```python
from build123d import *

# Parameters (mm, degrees)
SKETCH8_W           = 84.5
SKETCH8_H           = 12
SKETCH8_R           = 2.456134815
BOSS_EXTRUDE4_DEPTH = 8
SKETCH9_R           = 3.5
CUT_EXTRUDE3_DEPTH  = 2
SKETCH10_W          = 6
SKETCH10_H          = 12
BOSS_EXTRUDE5_DEPTH = 48
SKETCH11_W          = 8
SKETCH11_H          = 3.4
BOSS_EXTRUDE6_DEPTH = 35
SKETCH12_R          = 2
CUT_EXTRUDE4_DEPTH  = 35
SKETCH13_R          = 1.310160124
CUT_EXTRUDE5_DEPTH  = 10


with BuildPart() as part:
    # Sketch8 → Boss-Extrude4 (new body)
    with BuildSketch(Plane.XY):
        with Locations((17.439173688, 7.621093459)):
            Rectangle(SKETCH8_W, SKETCH8_H)
        with Locations((-18.810826312, 7.621093459)):
            Circle(SKETCH8_R, mode=Mode.SUBTRACT)
        with Locations((15.689173688, 7.621093459)):
            Circle(SKETCH8_R, mode=Mode.SUBTRACT)
    extrude(amount=BOSS_EXTRUDE4_DEPTH)

    # Sketch9 → Cut-Extrude3 (cut)
    with BuildSketch(Plane(origin=(0, 0, 0), x_dir=(-1, 0, 0), z_dir=(0, 0, -1))):
        with Locations((-15.689173688, 7.621093459)):
            Circle(SKETCH9_R)
        with Locations((18.810826312, 7.621093459)):
            Circle(SKETCH9_R)
    extrude(amount=-CUT_EXTRUDE3_DEPTH, mode=Mode.SUBTRACT)

    # Sketch10 → Boss-Extrude5 (add)
    with BuildSketch(Plane.XY.offset(8)):
        with Locations((56.689173688, 7.621093459)):
            Rectangle(SKETCH10_W, SKETCH10_H)
    extrude(amount=BOSS_EXTRUDE5_DEPTH)

    # Sketch11 → Boss-Extrude6 (add)
    with BuildSketch(Plane(origin=(59.689173688, 0, 0), x_dir=(0, 0, -1), z_dir=(1, 0, 0))):
        with Locations((-4, 3.321093459)):
            Rectangle(SKETCH11_W, SKETCH11_H)
        with Locations((-52, 3.321093459)):
            Rectangle(SKETCH11_W, SKETCH11_H)
    extrude(amount=BOSS_EXTRUDE6_DEPTH)

    # Sketch12 → Cut-Extrude4 (cut)
    with BuildSketch(Plane(origin=(0, 5.021093459, 0), x_dir=(1, 0, 0), z_dir=(0, 1, 0))):
        with Locations(Location((72.689173688, -3.25, 0), (0, 0, 180))):
            Circle(SKETCH12_R)
        with Locations(Location((82.689173688, -3.25, 0), (0, 0, 180))):
            Circle(SKETCH12_R)
        with Locations(Location((72.689173688, -52.75, 0), (0, 0, 180))):
            Circle(SKETCH12_R)
        with Locations(Location((82.689173688, -52.75, 0), (0, 0, 180))):
            Circle(SKETCH12_R)
    extrude(amount=-CUT_EXTRUDE4_DEPTH, mode=Mode.SUBTRACT)

    # Sketch13 → Cut-Extrude5 (cut)
    with BuildSketch(Plane(origin=(0, 0, 0), x_dir=(-1, 0, 0), z_dir=(0, 0, -1))):
        with Locations((1.505343306, 7.621093459)):
            Circle(SKETCH13_R)
    extrude(amount=-CUT_EXTRUDE5_DEPTH, mode=Mode.SUBTRACT)


solid = part.part
```
Here's how the part is built. I have some questions about the finished solid (model axes, mm). A direction names the side the tool comes from. Coordinates: 2 decimals unless noted, no trailing zeros. Write each loop counter-clockwise with the first axis right and the second up, starting at its lowest first coordinate (ties: lowest second). Pieces come first, ordered by that corner, then holes. Notation, with made-up numbers: (60.5, 0.5) -> (95.5, 0.5) arc R15 cw to (95.5, 20.5) -> close; hole circle Ø7 at (-35, 35). An arc over 180 degrees is marked (long way). Use a Markdown table: item, result. Add a question column.
(1) If we section it at B-B, the plane z = 3.25: Write out the boundary of the cut face in (x, y), and give its area (3 significant figures).
(2) For faces 5 (the cylindrical face through (12.35, 8.67, 0.99)), 6 (the flat face through (77, 5.021, 52)), 7 (the flat face through (77, 3, 48)), 8 (the flat face through (53.689, 8, 32)), which set-ups out of +Z, -Z, +X, -X, +Y, -Y let a thin tool reach every point of the face, with its end or its side?
(3) I'm going to push flat-ended pins straight in: P1, Ø6, axis at y = 5.5, z = 28, coming from the -X side; P2, Ø2.5, axis at x = 78, z = 3, coming from the +Y side; P3, Ø3.5, axis at x = 8.5, y = 8, coming from the +Z side. Where does each tip first touch, or does it pass through?
(4) If we section it at C-C, the plane x = 65.5: Write out the boundary of the cut face in (y, z).
(5) We'd pull the mould along X, two halves only. Please class faces 1 (the flat face through (94.689, 3, 4)), 2 (the cylindrical face through (-22.15, 8.67, 0.99)), 3 (the flat face through (-24.811, 8, 4)), 4 (the flat face through (21, 8, 0)): +X half, -X half, draft (parallel to the pull), parting line (faces both ways), or undercut.
(6) Please list where these lines run through material, in increasing order: line 1 (Z direction, x = 76, y = 4.25); line 2 (Z direction, x = 25, y = 12); line 3 (X direction, y = 3.25, z = 29).
(7) If we section it at A-A, the plane z = 52.75: Write out the boundary of the cut face in (x, y), and give its area (3 significant figures).
(8) If we section it at D-D, the plane y = 3: Write out the boundary of the cut face in (x, z).
Outcome:
| question | item | result |
|---|---|---|
| 1 | outline | (-24.81, 1.62) -> (70.69, 1.62) -> (70.69, 5.02) -> (59.69, 5.02) -> (59.69, 13.62) -> (-24.81, 13.62) -> close; (74.69, 1.62) -> (80.69, 1.62) -> (80.69, 5.02) -> (74.69, 5.02) -> close; (84.69, 1.62) -> (94.69, 1.62) -> (94.69, 5.02) -> (84.69, 5.02) -> close; hole circle Ø4.91 at (-18.81, 7.62); hole circle Ø2.62 at (-1.51, 7.62); hole circle Ø4.91 at (15.69, 7.62) |
| 1 | area | 1,060 mm^2 |
| 2 | face 5 | -Z |
| 2 | face 6 | +Z, -Z, +X, +Y |
| 2 | face 7 | +X, +Y, -Y |
| 2 | face 8 | +Z, -X, +Y, -Y |
| 3 | P1 | stops at x = 53.69 |
| 3 | P2 | stops at y = 5.02 |
| 3 | P3 | stops at z = 8 |
| 4 | outline | (1.62, 0) -> (5.02, 0) -> (5.02, 8) -> (1.62, 8) -> close; (1.62, 48) -> (5.02, 48) -> (5.02, 56) -> (1.62, 56) -> close |
| 5 | face 1 | +X half |
| 5 | face 2 | undercut |
| 5 | face 3 | -X half |
| 5 | face 4 | draft |
| 6 | line 1 | z = 0 to 8, 48 to 56 |
| 6 | line 2 | z = 0 to 8 |
| 6 | line 3 | x = 53.69 to 59.69 |
| 7 | outline | (53.69, 1.62) -> (70.69, 1.62) -> (70.69, 5.02) -> (59.69, 5.02) -> (59.69, 13.62) -> (53.69, 13.62) -> close; (74.69, 1.62) -> (80.69, 1.62) -> (80.69, 5.02) -> (74.69, 5.02) -> close; (84.69, 1.62) -> (94.69, 1.62) -> (94.69, 5.02) -> (84.69, 5.02) -> close |
| 7 | area | 164 mm^2 |
| 8 | outline | (-24.81, 0) -> (94.69, 0) -> (94.69, 8) -> (59.69, 8) -> (59.69, 48) -> (94.69, 48) -> (94.69, 56) -> (53.69, 56) -> (53.69, 8) -> (-24.81, 8) -> close; hole circle Ø4 at (72.69, 3.25); hole circle Ø4 at (72.69, 52.75); hole circle Ø4 at (82.69, 3.25); hole circle Ø4 at (82.69, 52.75) |
